For this review, take the finished solid that the model builds, in its own axes (mm). A direction names the side the tool comes from. Coordinates: 2 decimals unless noted, no trailing zeros. Loops run counter-clockwise (first coordinate to the right, second up) from the corner with the lowest first, then second, coordinate; pieces in that order, holes last. Notation, with made-up numbers: (30, 42.25) - (59, 42.25) arc R34 ccw to (59, 77.25) - close; hole circle Ø6 at (49.25, 35.25). An arc over 180 degrees is marked (long way). Use one line per item in the form item = value. Start each with the question number.
1. Machinability: for faces 1 (the face through (108, 55.647, 13)), 2 (the face through (76.167, 30, 13)), 3 (the face through (-76, 93.747, 13)), which of the approach directions +Z, -Z, +X, -X, +Y, -Y give a long, thin tool a straight path to every point of the face, cutting with its end or side? Answer none if there is none.
2. To check wall thickness, follow probe 1 along Y at (x, z) = (36, 18); probe 2 along X at (y, z) = (27, 23.5); probe 3 along X at (y, z) = (30.5, 9.5). State the ranges of each line that lie inside material, in increasing order.
3. Add section C-C on x = 99. Give the boundary of the cut face in (y, z).
4. Add section A-A on y = 34.5. Give the boundary of the cut face in (x, z), and give its area (3 significant figures).
5. Add section D-D on y = 69. Give the boundary of the cut face in (x, z), and give its area (3 significant figures).
6. Draft analysis for pull direction X (two halves, no side actions). For faces 4 (the face through (17, -58.653, 13)), 5 (the face through (-23.6, 82.29, 12.52)), 6 (the face through (39, 17.547, 13)), 7 (the face through (79.986, 52.025, 12.522)), state which applies: +X half, -X half, draft (parallel to the pull), parting line (faces both ways), or undercut.
7. For pin 1 Ø12 at (y, z) = (57.5, 19) entering from +X; pin 2 Ø7.5 at (x, z) = (48, 17) entering from +Y, all flat-tipped, find the tip position at first contact; note any pin that passes through.
8. Add section B-B on z = 11. Give the boundary of the cut face in (x, y).
```python
from build123d import *

# Parameters (mm, degrees)
F1_DEPTH = 25.4


with BuildPart() as f1:
    # F0 (on Top) → F1 (new body)
    with BuildSketch(Plane.XY):
        with BuildLine():
            Line((-114.333168, 81.04653), (-114.333168, -58.65347))
            Line((-114.333168, -58.65347), (152.366832, -58.65347))
            ThreePointArc((152.366832, -58.65347), (161.347088, -54.933726), (165.066832, -45.95347))
            Line((165.066832, -45.95347), (165.066832, 17.54653))
            ThreePointArc((165.066832, 17.54653), (153.907601, 44.487298), (126.966832, 55.64653))
            Line((126.966832, 55.64653), (88.866832, 55.64653))
            ThreePointArc((88.866832, 55.64653), (79.886576, 51.926786), (76.166832, 42.94653))
            Line((76.166832, 42.94653), (76.166832, 17.54653))
            Line((76.166832, 17.54653), (-0.033168, 17.54653))
            ThreePointArc((-0.033168, 17.54653), (-9.013424, 21.266274), (-12.733168, 30.24653))
            Line((-12.733168, 30.24653), (-12.733168, 55.64653))
            ThreePointArc((-12.733168, 55.64653), (-23.892399, 82.587298), (-50.833168, 93.74653))
            Line((-50.833168, 93.74653), (-101.633168, 93.74653))
            ThreePointArc((-101.633168, 93.74653), (-110.613424, 90.026786), (-114.333168, 81.04653))
        make_face()
    extrude(amount=F1_DEPTH)


solid = f1.part
```
Conclusion:
q1.face_1 = +Z, -Z, +X, +Y
q1.face_2 = +Z, -Z, +Y
q1.face_3 = +Z, -Z, +X, -X, +Y
q2.probe_1 = -58.65 to 17.55
q2.probe_2 = -114.33 to -12.31, 76.17 to 163.88
q2.probe_3 = -114.33 to -12.73, 76.17 to 162.8
q3.outline = (-58.65, 0) - (55.65, 0) - (55.65, 25.4) - (-58.65, 25.4) - close
q4.outline = (-114.33, 0) - (-12.73, 0) - (-12.73, 25.4) - (-114.33, 25.4) - close; (76.17, 0) - (161.09, 0) - (161.09, 25.4) - (76.17, 25.4) - close
q4.area = 4,740 mm^2
q5.outline = (-114.33, 0) - (-15.15, 0) - (-15.15, 25.4) - (-114.33, 25.4) - close
q5.area = 2,520 mm^2
q6.face_4 = draft
q6.face_5 = +X half
q6.face_6 = undercut
q6.face_7 = undercut
q7.pin_1 = 144.25
q7.pin_2 = 17.55
q8.outline = (-114.33, -58.65) - (152.37, -58.65) arc R12.7 ccw to (165.07, -45.95) - (165.07, 17.55) arc R38.1 ccw to (126.97, 55.65) - (88.87, 55.65) arc R12.7 ccw to (76.17, 42.95) - (76.17, 17.55) - (-0.03, 17.55) arc R12.7 cw to (-12.73, 30.25) - (-12.73, 55.65) arc R38.1 ccw to (-50.83, 93.75) - (-101.63, 93.75) arc R12.7 ccw to (-114.33, 81.05) - close
